from build123d import *

# Parameters (mm, degrees)
F0_W     = 31.75
F0_H     = 31.75
F1_DEPTH = 41.275
F2_W     = 25.4
F2_H     = 25.4
F3_DEPTH = 50.8
F4_R     = 4.7625
F5_DEPTH = 28.576


with BuildPart() as f1:
    # F0 (on Top) → F1 (new body)
    with BuildSketch(Plane.XY):
        with Locations((15.875, 15.875)):
            Rectangle(F0_W, F0_H)
    extrude(amount=F1_DEPTH)

    # F2 (on face) → F3 (join)
    with BuildSketch(Plane(origin=(0, 0, 0), x_dir=(1, 0, 0), z_dir=(0, 0, -1))):
        with Locations((15.875, -15.875)):
            Rectangle(F2_W, F2_H)
    extrude(amount=F3_DEPTH)

    # F4 (on face) → F5 (cut, through all)
    with BuildSketch(Plane.XZ.offset(-3.175)):
        with Locations((15.875, -31.75)):
            Circle(F4_R)
    extrude(amount=-F5_DEPTH, mode=Mode.SUBTRACT)


solid = f1.part
Can you work these out from the model? Positions are in its coordinate system, mm. A direction names the side the tool comes from. Give positions to 0.01 mm unless a question says otherwise; leave off trailing zeros. Loops run counter-clockwise (first coordinate to the right, second up) from the corner with the lowest first, then second, coordinate; pieces in that order, holes last. Notation, with made-up numbers: M -10,11 L 49,11 A29 cw 49,48 Z; hole C 15,88 d8. An arc over 180 degrees is marked long. One line per item, written item: value. Start each with the question number.
1) On a 3-axis mill with a long thin cutter (end or side, diameter ignored), from which of +Z, -Z, +X, -X, +Y, -Y can I reach the whole of each face in a straight line? I mean faces 1 (the face through (28.575, 16, -25)), 2 (the face through (16, 28.575, -25)), 3 (the face through (31.75, 16, 20)). Say none if no direction works.
2) I'm going to push flat-ended pins straight in: pin 1 (12.5 mm diameter, centred on y = 15.5, z = -25.5, fed in from +X) (3 decimals); pin 2 (7.5 mm diameter, centred on x = 19.5, z = -29.5, fed in from +Y) (3 decimals); pin 3 (5 mm diameter, centred on x = 9.5, z = 16.5, fed in from -Y); pin 4 (1.5 mm diameter, centred on y = 11, z = -38, fed in from -X) (3 decimals). Where does each tip first touch, or does it pass through?
3) If we section it at C-C, the plane x = 13.5: Write out the boundary of the cut face in (y, z) (3 decimals).
4) If I drill on line 1 (Z direction, x = 16, y = 25) (3 decimals); line 2 (Z direction, x = 2, y = 16) (3 decimals); line 3 (X direction, y = 12, z = -18.5) (3 decimals), over which ranges is the centre line in solid material (lowest first)? Write a range as [from, to].
5) Thinking about a two-plate mould opening in X: for faces 4 (the face through (16, 3.175, -25)), 5 (the face through (11.117, 15.697, -31.541)), 6 (the face through (3.175, 16, -25)), which applies, +X half, -X half, draft (parallel to the pull), parting line (faces both ways), or undercut?
6) If we section it at D-D, the plane x = 25.5: Write out the boundary of the cut face in (y, z) (3 decimals).
7) If we section it at A-A, the plane z = -31.75: Write out the boundary of the cut face in (x, y) (1 decimal).
Completed:
1. face 1: -Z, +X, +Y, -Y
1. face 2: -Z, +X, -X, +Y
1. face 3: +Z, -Z, +X, +Y, -Y
2. pin 1: stops at x = 28.575
2. pin 2: stops at y = 28.575
2. pin 3: stops at y = 0
2. pin 4: stops at x = 3.175
3. outline: M 0,0 L 3.175,0 L 3.175,-27.622 L 28.575,-27.622 L 28.575,0 L 31.75,0 L 31.75,41.275 L 0,41.275 Z; M 3.175,-50.8 L 28.575,-50.8 L 28.575,-35.878 L 3.175,-35.878 Z
4. line 1: z = [-50.8, -36.511], [-26.989, 41.275]
4. line 2: z = [0, 41.275]
4. line 3: x = [3.175, 28.575]
5. face 4: draft
5. face 5: undercut
5. face 6: -X half
6. outline: M 0,0 L 3.175,0 L 3.175,-50.8 L 28.575,-50.8 L 28.575,0 L 31.75,0 L 31.75,41.275 L 0,41.275 Z
7. outline: M 3.2,3.2 L 11.1,3.2 L 11.1,28.6 L 3.2,28.6 Z; M 20.6,3.2 L 28.6,3.2 L 28.6,28.6 L 20.6,28.6 Z
